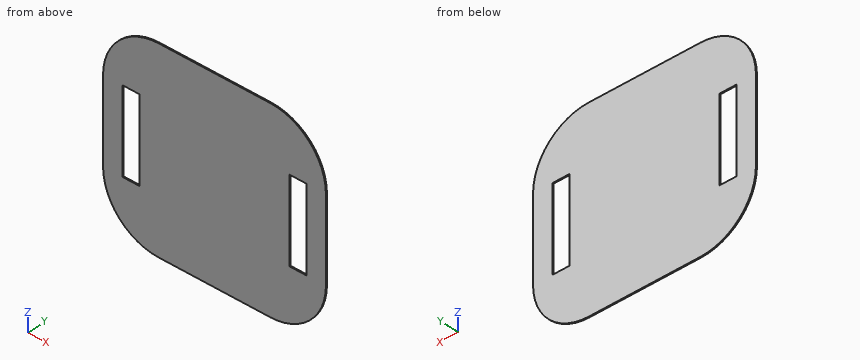
```python
from build123d import *

# Parameters (mm, degrees)
SKETCH2_W           = 400
SKETCH2_H           = 350
BASE_FLANGE1_DEPTH  = 2
CUT_EXTRUDE1_REACH  = 267.761
SKETCH7_W           = 30
SKETCH7_H           = 150
BREAK_CORNER1_DEPTH = 2


# Read off the part's stored shape, not the designer's step: Break-Corner1
# Sheet-metal steps are written as plain solids
with BuildPart() as part:
    # Sketch2 → Base-Flange1 (new body)
    with BuildSketch(Plane(origin=(0, 0, 0), x_dir=(1, 0, 0), z_dir=(0, 1, 0))):
        Rectangle(SKETCH2_W, SKETCH2_H)
    extrude(amount=BASE_FLANGE1_DEPTH)

    # Sketch7 → Cut-Extrude1 (cut, up to next)
    with BuildSketch(Plane(origin=(0, 2, 0), x_dir=(1, 0, 0), z_dir=(0, 1, 0)), mode=Mode.PRIVATE) as cut_extrude1_sk1:
        with Locations((-150, 0)):
            Rectangle(SKETCH7_W, SKETCH7_H)
    cut_extrude1_tool1 = extrude(cut_extrude1_sk1.sketch, amount=-CUT_EXTRUDE1_REACH, mode=Mode.PRIVATE) & part.part
    # Sketch7 → Cut-Extrude1 (cut, up to next)
    with BuildSketch(Plane(origin=(0, 2, 0), x_dir=(1, 0, 0), z_dir=(0, 1, 0)), mode=Mode.PRIVATE) as cut_extrude1_sk2:
        with Locations((150, 0)):
            Rectangle(SKETCH7_W, SKETCH7_H)
    cut_extrude1_tool2 = extrude(cut_extrude1_sk2.sketch, amount=-CUT_EXTRUDE1_REACH, mode=Mode.PRIVATE) & part.part
    add(cut_extrude1_tool1.solids().sort_by_distance((-150, 2, 0))[0], mode=Mode.SUBTRACT)
    add(cut_extrude1_tool2.solids().sort_by_distance((150, 2, 0))[0], mode=Mode.SUBTRACT)

    # Break-Corner1 outline → Break-Corner1 (cut)
    with BuildSketch(Plane(origin=(0, 0, 0), x_dir=(1, 0, 0), z_dir=(0, 1, 0))):
        with BuildLine():
            Line((-200, 175), (-200, 75))
            ThreePointArc((-200, 75), (-170.710678119, 145.710678119), (-100, 175))
            Line((-100, 175), (-200, 175))
        make_face()
        with BuildLine():
            ThreePointArc((-100, -175), (-170.710678119, -145.710678119), (-200, -75))
            Line((-200, -75), (-200, -175))
            Line((-200, -175), (-100, -175))
        make_face()
        with BuildLine():
            Line((200, 175), (100, 175))
            ThreePointArc((100, 175), (170.710678119, 145.710678119), (200, 75))
            Line((200, 75), (200, 175))
        make_face()
        with BuildLine():
            ThreePointArc((200, -75), (170.710678119, -145.710678119), (100, -175))
            Line((100, -175), (200, -175))
            Line((200, -175), (200, -75))
        make_face()
    extrude(amount=BREAK_CORNER1_DEPTH, mode=Mode.SUBTRACT)


solid = part.part
```
Part model, mm, in its own coordinate system. Round coordinates to 2 decimals unless told otherwise and drop trailing zeros. Write each loop counter-clockwise with the first axis right and the second up, starting at its lowest first coordinate (ties: lowest second). Pieces come first, ordered by that corner, then holes. Notation, with made-up numbers: (-31.5, 16) -> (-1.5, 16) arc R6 cw to (-1.5, 21) -> close; hole circle Ø1 at (41.5, -27.5). An arc over 180 degrees is marked (long way). Return JSON: item names as keys, results as strings. Group by question number.
Q1. Pin check, flat tip, straight feed: pin 1 (1 mm diameter, centred on x = -146.5, y = 1, fed in from +Z). Stop position of the tip, or through.
Q2. Saw through at B-B on z = -70.5. Write the cut outline in (x, y), plus the area to 3 significant figures.
Q3. Saw through at A-A on y = 1.3. Write the cut outline in (x, z), plus the area to 3 significant figures.
Q4. Saw through at D-D on x = -149. Write the cut outline in (y, z).
Q5. Saw through at C-C on x = 158.5. Write the cut outline in (y, z), plus the area to 3 significant figures.
Q6. Probe L1, parallel to X at y = 0.6, z = -18; L2, parallel to Z at x = -101, y = 1.4 (3 decimals); L3, parallel to Z at x = 157, y = 0.35. List the from-to ranges inside material, lowest first. Write a range as [from, to].
Answer:
{
 "1": {"pin 1": "z = 163.79"},
 "2": {"outline": "(-200, 0) -> (-165, 0) -> (-165, 2) -> (-200, 2) -> close; (-135, 0) -> (135, 0) -> (135, 2) -> (-135, 2) -> close; (165, 0) -> (200, 0) -> (200, 2) -> (165, 2) -> close", "area": "680 mm2"},
 "3": {"outline": "(-200, -75) arc R100 ccw to (-100, -175) -> (100, -175) arc R100 ccw to (200, -75) -> (200, 75) arc R100 ccw to (100, 175) -> (-100, 175) arc R100 ccw to (-200, 75) -> close; hole (-165, -75) -> (-135, -75) -> (-135, 75) -> (-165, 75) -> close; hole (135, -75) -> (165, -75) -> (165, 75) -> (135, 75) -> close", "area": "122,000 mm2"},
 "4": {"outline": "(0, -162.17) -> (2, -162.17) -> (2, -75) -> (0, -75) -> close; (0, 75) -> (2, 75) -> (2, 162.17) -> (0, 162.17) -> close"},
 "5": {"outline": "(0, -156.1) -> (2, -156.1) -> (2, -75) -> (0, -75) -> close; (0, 75) -> (2, 75) -> (2, 156.1) -> (0, 156.1) -> close", "area": "324 mm2"},
 "6": {"L1": "[-200, -165], [-135, 135], [165, 200]", "L2": "[-174.995, 174.995]", "L3": "[-157.16, -75], [75, 157.16]"}
}
